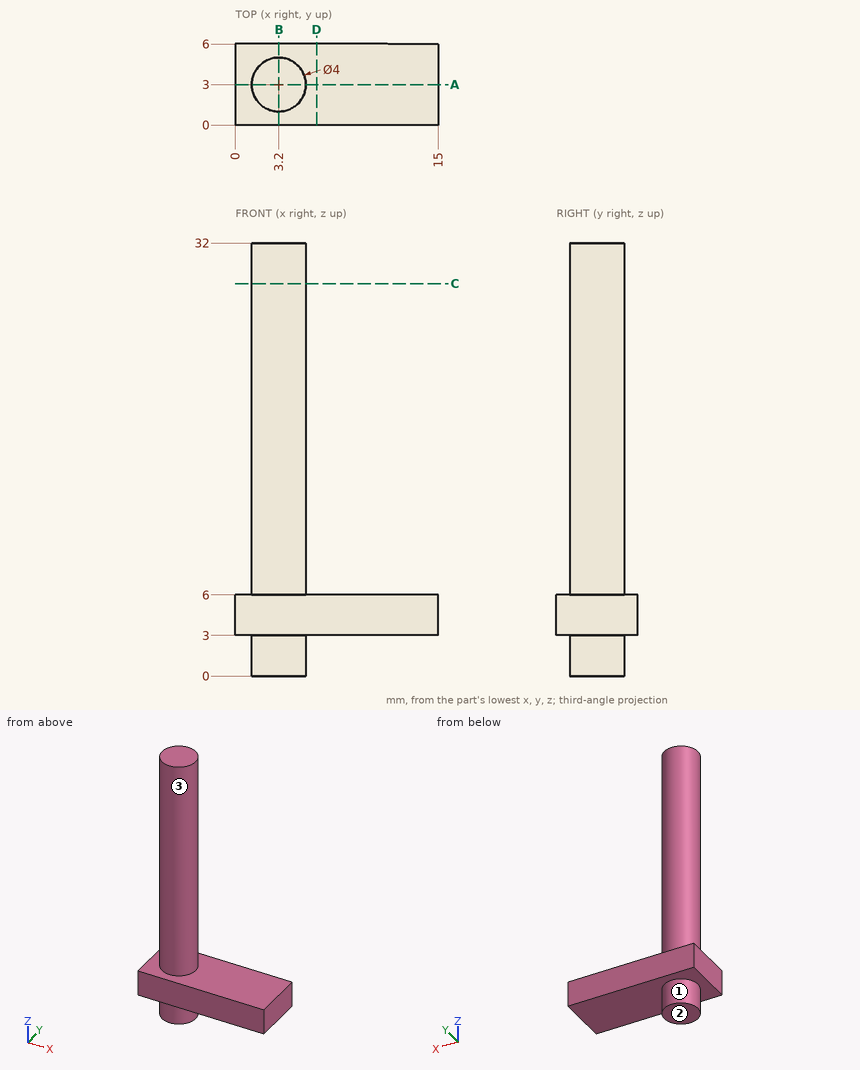
Print and shaded views of the part. All mm, measured from the part's lowest x, y and z. A direction names the side the tool comes from. Coordinates: 2 decimals unless noted, no trailing zeros. Order: outer loops, then holes, each group sorted by start corner. A loop starts at its lowest first (then second) coordinate and runs counter-clockwise, first axis right, second up. Notation, with made-up numbers: (-2, -33) -> (8, -33) arc R33 cw to (8, 3) -> close; hole circle Ø6 at (-7.75, 82). An arc over 180 degrees is marked (long way). Use one line per item in the form item = value. Start each with the question number.
1) Band-saw the part on B-B on x = 3.2. Give the cut face in (y, z).
2) Drill centre lines: L1, parallel to X at y = 3, z = 24.5; L2, parallel to Z at x = 8, y = 3; L3, parallel to X at y = 4.5, z = 13. Where is each one in solid material? Low to high. Write a range as [from, to].
3) Drop flat-ended pins along their axis: pin 1 (6 mm diameter, centred on x = 6.5, z = 25.5, fed in from +Y); pin 2 (8 mm diameter, centred on x = 12.5, z = 20, fed in from +Y); pin 3 (1.5 mm diameter, centred on y = 4, z = 23, fed in from -X); pin 4 (2 mm diameter, centred on x = 12, y = 2, fed in from -Z). Give the stop position or say it passes through.
4) Tool access for the marked faces 1, 2 and 3: list every direction of +Z, -Z, +X, -X, +Y, -Y with a clear straight run to the whole face (end or side of a thin tool).
5) Band-saw the part on A-A on y = 3. Give the cut face in (x, z), then the cut area to 3 significant figures.
6) Band-saw the part on C-C on z = 29. Give the cut face in (x, y), then the cut area to 3 significant figures.
7) Band-saw the part on D-D on x = 6. Give the cut face in (y, z), then the cut area to 3 significant figures.
Entries:
q1.outline = (0, 3) -> (1, 3) -> (1, 0) -> (5, 0) -> (5, 3) -> (6, 3) -> (6, 6) -> (5, 6) -> (5, 32) -> (1, 32) -> (1, 6) -> (0, 6) -> close
q2.L1 = [1.2, 5.2]
q2.L2 = [3, 6]
q2.L3 = [1.88, 4.52]
q3.pin_1 = 4.98
q3.pin_2 = through
q3.pin_3 = 1.22
q3.pin_4 = 3
q4.face_1 = -Z
q4.face_2 = -Z, +X, -X, +Y, -Y
q4.face_3 = +Z
q5.outline = (0, 3) -> (1.2, 3) -> (1.2, 0) -> (5.2, 0) -> (5.2, 3) -> (15, 3) -> (15, 6) -> (5.2, 6) -> (5.2, 32) -> (1.2, 32) -> (1.2, 6) -> (0, 6) -> close
q5.area = 161 mm2
q6.outline = circle Ø4 at (3.2, 3)
q6.area = 12.6 mm2
q7.outline = (0, 3) -> (6, 3) -> (6, 6) -> (0, 6) -> close
q7.area = 18.0 mm2
